from build123d import *

# Parameters (mm, degrees)
SKETCH1_R           = 1.8
BOSS_EXTRUDE1_DEPTH = 6
BOSS_EXTRUDE2_DEPTH = 40
CUT_EXTRUDE1_REACH  = 94.7
SKETCH3_W           = 20
SKETCH3_H           = 12.5
SKETCH4_R           = 3.25
CUT_EXTRUDE2_DEPTH  = 19
CUT_EXTRUDE3_REACH  = 102.286
CUT_EXTRUDE4_START  = -7
CUT_EXTRUDE4_DEPTH  = 26
SKETCH7_W           = 27
SKETCH7_H           = 36
CUT_EXTRUDE5_DEPTH  = 6
CUT_EXTRUDE6_REACH  = 95.13
SKETCH9_W           = 27
SKETCH9_H           = 32
CUT_EXTRUDE7_DEPTH  = 2
CUT_EXTRUDE10_DEPTH = 101.285841473
FILLET1_R           = 3
CUT_EXTRUDE11_DEPTH = 6
SKETCH12_W          = 8
SKETCH12_H          = 6
SKETCH12_W_2        = 10
BOSS_EXTRUDE3_DEPTH = 3
SKETCH13_R          = 2
CUT_EXTRUDE12_DEPTH = 6


with BuildPart() as part:
    # Sketch1 → Boss-Extrude1 (new body)
    with BuildSketch(Plane(origin=(0, 0, 0), x_dir=(1, 0, 0), z_dir=(0, 1, 0))):
        Polygon((68.5, 20), (68.5, 7.5), (88.5, 7.5), (88.5, -7.5), (68.5, -7.5), (68.5, -20), (-68.5, -20), (-68.5, -7.5), (-88.5, -7.5), (-88.5, 7.5), (-68.5, 7.5), (-68.5, 20), align=None)
        with Locations(Location((-78.5, 0, 0), (0, 0, 270))):
            Circle(SKETCH1_R, mode=Mode.SUBTRACT)
        with Locations(Location((-58.5, 8.5, 0), (0, 0, 270))):
            Circle(SKETCH1_R, mode=Mode.SUBTRACT)
        with Locations(Location((-58.5, -8.5, 0), (0, 0, 270))):
            Circle(SKETCH1_R, mode=Mode.SUBTRACT)
        with Locations(Location((58.5, -8.5, 0), (0, 0, 90))):
            Circle(SKETCH1_R, mode=Mode.SUBTRACT)
        with Locations(Location((78.5, 0, 0), (0, 0, 90))):
            Circle(SKETCH1_R, mode=Mode.SUBTRACT)
        with Locations(Location((58.5, 8.5, 0), (0, 0, 90))):
            Circle(SKETCH1_R, mode=Mode.SUBTRACT)
    extrude(amount=BOSS_EXTRUDE1_DEPTH)

    # Sketch2 → Boss-Extrude2 (add)
    with BuildSketch(Plane(origin=(0, 0, -20), x_dir=(-1, 0, 0), z_dir=(0, 0, -1))):
        Polygon((-88.5, 6), (88.5, 6), (88.5, 9), (58.5, 18), (48.5, 25), (-48.5, 25), (-58.5, 18), (-88.5, 9), align=None)
    extrude(amount=-BOSS_EXTRUDE2_DEPTH)

    # Sketch3 → Cut-Extrude1 (cut, up to next)
    with BuildSketch(Plane.XZ.offset(-6), mode=Mode.PRIVATE) as cut_extrude1_sk1:
        with Locations((-78.5, 13.75)):
            Rectangle(SKETCH3_W, SKETCH3_H)
    cut_extrude1_tool1 = extrude(cut_extrude1_sk1.sketch, amount=-CUT_EXTRUDE1_REACH, mode=Mode.PRIVATE) & part.part
    # Sketch3 → Cut-Extrude1 (cut, up to next)
    with BuildSketch(Plane.XZ.offset(-6), mode=Mode.PRIVATE) as cut_extrude1_sk2:
        with Locations((-78.5, -13.75)):
            Rectangle(SKETCH3_W, SKETCH3_H)
    cut_extrude1_tool2 = extrude(cut_extrude1_sk2.sketch, amount=-CUT_EXTRUDE1_REACH, mode=Mode.PRIVATE) & part.part
    # Sketch3 → Cut-Extrude1 (cut, up to next)
    with BuildSketch(Plane.XZ.offset(-6), mode=Mode.PRIVATE) as cut_extrude1_sk3:
        with Locations((78.5, 13.75)):
            Rectangle(SKETCH3_W, SKETCH3_H)
    cut_extrude1_tool3 = extrude(cut_extrude1_sk3.sketch, amount=-CUT_EXTRUDE1_REACH, mode=Mode.PRIVATE) & part.part
    # Sketch3 → Cut-Extrude1 (cut, up to next)
    with BuildSketch(Plane.XZ.offset(-6), mode=Mode.PRIVATE) as cut_extrude1_sk4:
        with Locations((78.5, -13.75)):
            Rectangle(SKETCH3_W, SKETCH3_H)
    cut_extrude1_tool4 = extrude(cut_extrude1_sk4.sketch, amount=-CUT_EXTRUDE1_REACH, mode=Mode.PRIVATE) & part.part
    add(cut_extrude1_tool1.solids().sort_by_distance((-78.5, 6, 13.75))[0], mode=Mode.SUBTRACT)
    add(cut_extrude1_tool2.solids().sort_by_distance((-78.5, 6, -13.75))[0], mode=Mode.SUBTRACT)
    add(cut_extrude1_tool3.solids().sort_by_distance((78.5, 6, 13.75))[0], mode=Mode.SUBTRACT)
    add(cut_extrude1_tool4.solids().sort_by_distance((78.5, 6, -13.75))[0], mode=Mode.SUBTRACT)

    # Sketch4 → Cut-Extrude2 (cut)
    with BuildSketch(Plane(origin=(0, 25, 0), x_dir=(1, 0, 0), z_dir=(0, 1, 0))):
        with Locations(Location((-58.5, 8.5, 0), (0, 0, 90))):
            Circle(SKETCH4_R)
        with Locations(Location((-78.5, 0, 0), (0, 0, 90))):
            Circle(SKETCH4_R)
        with Locations(Location((-58.5, -8.5, 0), (0, 0, 90))):
            Circle(SKETCH4_R)
        with Locations(Location((58.5, 8.5, 0), (0, 0, 90))):
            Circle(SKETCH4_R)
        with Locations(Location((58.5, -8.5, 0), (0, 0, 90))):
            Circle(SKETCH4_R)
        with Locations(Location((78.5, 0, 0), (0, 0, 180))):
            Circle(SKETCH4_R)
    extrude(amount=-CUT_EXTRUDE2_DEPTH, mode=Mode.SUBTRACT)

    # Sketch5 → Cut-Extrude3 (cut, up to next)
    with BuildSketch(Plane(origin=(0, 0, -20), x_dir=(-1, 0, 0), z_dir=(0, 0, -1)), mode=Mode.PRIVATE) as cut_extrude3_sk1:
        Polygon((48.5, 0), (30, 15), (-30, 15), (-48.5, 0), align=None)
    cut_extrude3_tool1 = extrude(cut_extrude3_sk1.sketch, amount=-CUT_EXTRUDE3_REACH, mode=Mode.PRIVATE) & part.part
    add(cut_extrude3_tool1.solids().sort_by_distance((0, 6.910828, -20))[0], mode=Mode.SUBTRACT)

    # Sketch6 → Cut-Extrude4 (cut)
    with BuildSketch(Plane(origin=(0, 0, -20), x_dir=(-1, 0, 0), z_dir=(0, 0, -1)).offset(CUT_EXTRUDE4_START)):
        Polygon((43.1, 4.378378378), (43.1, 20.378378378), (-53.9, 20.378378378), (-53.9, 0), (-48.5, 0), (-30, 15), (30, 15), align=None)
    extrude(amount=-CUT_EXTRUDE4_DEPTH, mode=Mode.SUBTRACT)

    # Sketch7 → Cut-Extrude5 (cut)
    with BuildSketch(Plane(origin=(0, 15, 0), x_dir=(-1, 0, 0), z_dir=(0, -1, 0))):
        with Locations((-5.5, 0)):
            Rectangle(SKETCH7_W, SKETCH7_H)
    extrude(amount=-CUT_EXTRUDE5_DEPTH, mode=Mode.SUBTRACT)

    # Sketch8 → Cut-Extrude6 (cut, up to next)
    with BuildSketch(Plane.XZ.offset(-21), mode=Mode.PRIVATE) as cut_extrude6_sk1:
        with BuildLine():
            Line((17, -18), (-6, -18))
            ThreePointArc((-6, -18), (-8, -16), (-6, -14))
            Line((-6, -14), (17, -14))
            ThreePointArc((17, -14), (19, -16), (17, -18))
        make_face()
    cut_extrude6_tool1 = extrude(cut_extrude6_sk1.sketch, amount=-CUT_EXTRUDE6_REACH, mode=Mode.PRIVATE) & part.part
    # Sketch8 → Cut-Extrude6 (cut, up to next)
    with BuildSketch(Plane.XZ.offset(-21), mode=Mode.PRIVATE) as cut_extrude6_sk2:
        with BuildLine():
            Line((17, 14), (-6, 14))
            ThreePointArc((-6, 14), (-8, 16), (-6, 18))
            Line((-6, 18), (17, 18))
            ThreePointArc((17, 18), (19, 16), (17, 14))
        make_face()
    cut_extrude6_tool2 = extrude(cut_extrude6_sk2.sketch, amount=-CUT_EXTRUDE6_REACH, mode=Mode.PRIVATE) & part.part
    add(cut_extrude6_tool1.solids().sort_by_distance((5.5, 21, -16))[0], mode=Mode.SUBTRACT)
    add(cut_extrude6_tool2.solids().sort_by_distance((5.5, 21, 16))[0], mode=Mode.SUBTRACT)

    # Sketch9 → Cut-Extrude7 (cut)
    with BuildSketch(Plane(origin=(0, 25, 0), x_dir=(1, 0, 0), z_dir=(0, 1, 0))):
        with Locations((5.5, 0)):
            Rectangle(SKETCH9_W, SKETCH9_H)
    extrude(amount=-CUT_EXTRUDE7_DEPTH, mode=Mode.SUBTRACT)

    # Sketch10 → Cut-Extrude10 (cut, through all)
    with BuildSketch(Plane(origin=(0, 0, -20), x_dir=(-1, 0, 0), z_dir=(0, 0, -1))):
        Polygon((43.1, 4.378378378), (30, 15), (43.1, 15), align=None)
    extrude(amount=-CUT_EXTRUDE10_DEPTH, mode=Mode.SUBTRACT)

    # Fillet1
    fillet1_edges = [part.edges().sort_by_distance(p)[0] for p in [
        (-43.1, 15, -16.5),
        (-43.1, 15, 16.5),
    ]]
    fillet(fillet1_edges, radius=FILLET1_R)

    # Sketch11 → Cut-Extrude11 (cut)
    with BuildSketch(Plane.XY.offset(20)):
        Polygon((25.5, 25), (48.5, 25), (58.5, 18), (68.5, 15), (68.5, 3), (52.633333333, 3), align=None)
        with BuildLine():
            Line((-68.5, 3), (-47.7, 3))
            Line((-47.7, 3), (-47.7, 13.5))
            ThreePointArc((-47.7, 13.5), (-46.528427125, 16.328427125), (-43.7, 17.5))
            Line((-43.7, 17.5), (-23.75, 17.5))
            Line((-23.75, 17.5), (-14.5, 25))
            Line((-14.5, 25), (-48.5, 25))
            Line((-48.5, 25), (-58.5, 18))
            Line((-58.5, 18), (-68.5, 15))
            Line((-68.5, 15), (-68.5, 3))
        make_face()
    cut_extrude11 = extrude(amount=-CUT_EXTRUDE11_DEPTH, mode=Mode.SUBTRACT)

    # Mirror1: Cut-Extrude11 across plane
    add(cut_extrude11.mirror(Plane(origin=(0, 0, 0), x_dir=(1, 0, 0), z_dir=(0, 0, -1))), mode=Mode.SUBTRACT)

    # Sketch12 → Boss-Extrude3 (add)
    with BuildSketch(Plane(origin=(0, 3, 0), x_dir=(1, 0, 0), z_dir=(0, 1, 0))):
        with Locations((-51.7, 17)):
            Rectangle(SKETCH12_W, SKETCH12_H)
        with Locations((-51.7, -17)):
            Rectangle(SKETCH12_W, SKETCH12_H)
        with Locations((53.5, -17)):
            Rectangle(SKETCH12_W_2, SKETCH12_H)
        with Locations((53.5, 17)):
            Rectangle(SKETCH12_W_2, SKETCH12_H)
    extrude(amount=BOSS_EXTRUDE3_DEPTH)

    # Sketch13 → Cut-Extrude12 (cut)
    with BuildSketch(Plane(origin=(0, 6, 0), x_dir=(1, 0, 0), z_dir=(0, 1, 0))):
        with Locations(Location((54.5, -17, 0), (0, 0, 270))):
            Circle(SKETCH13_R)
        with Locations(Location((54.5, 17, 0), (0, 0, 270))):
            Circle(SKETCH13_R)
        with Locations(Location((-51.7, 17, 0), (0, 0, 270))):
            Circle(SKETCH13_R)
        with Locations(Location((-51.7, -17, 0), (0, 0, 270))):
            Circle(SKETCH13_R)
    extrude(amount=-CUT_EXTRUDE12_DEPTH, mode=Mode.SUBTRACT)


solid = part.part
CAD build for the part. Positions are in the model's coordinates, mm. A direction names the side the tool comes from. Give positions to 0.01 mm unless a question says otherwise; leave off trailing zeros. Loops run counter-clockwise (first coordinate to the right, second up) from the corner with the lowest first, then second, coordinate; pieces in that order, holes last. Notation, with made-up numbers: M 16.25,-26 L 43.25,-26 A26 ccw 43.25,-11 Z; hole C -17.5,67 d10. An arc over 180 degrees is marked long. Write each question's results on one line, items separated by ' | '.
Q1. Probe probe 1 along X at (y, z) = (8, 0); probe 2 along X at (y, z) = (14.5, 8.5); probe 3 along Z at (x, y) = (-78.5, 1.55). List the from-to ranges inside material, lowest first.
Geometry check:
probe 1: x = -88.5 to -81.75, -75.25 to -43.1, 53.9 to 75.25, 81.75 to 88.5 | probe 2: x = -68.5 to -61.75, -55.25 to -43.1, 53.9 to 55.25, 61.75 to 68.5 | probe 3: z = -7.5 to -1.8, 1.8 to 7.5
Q2. Band-saw the part on A-A on x = -78.5. Write the cut outline in (y, z).
Geometry check:
outline: M 0,-7.5 L 12,-7.5 L 12,-3.25 L 6,-3.25 L 6,-1.8 L 0,-1.8 Z; M 0,1.8 L 6,1.8 L 6,3.25 L 12,3.25 L 12,7.5 L 0,7.5 Z
Q3. Flat gauge pins, fed straight in: P1, Ø1.5, axis at y = 5, z = -16.5, coming from the +X side; P2, Ø5, axis at x = -52, z = -17, coming from the +Y side; P3, Ø2, axis at x = 32.5, y = 11, coming from the +Z side; P4, Ø3, axis at x = 64, z = -11.5, coming from the +Y side. Where does each tip first touch, or does it go through?
Geometry check:
P1: stops at x = 58.5 | P2: stops at y = 6 | P3: passes through | P4: stops at y = 16.8
Q4. Mould opens along Z. For faces 6 (the face through (39.12, 7.605, -16.549)), 7 (the face through (0.3, 15.3, 20)), 8 (the face through (55.278, 11.671, 8.923)) say: pulls with the +Z half, pulls with the -Z half, needs draft (parallel to the pull), parting line crosses it, or undercut.
Geometry check:
face 6: needs draft | face 7: pulls with the +Z half | face 8: undercut
Q5. Which spindle directions (+Z, -Z, +X, -X, +Y, -Y) get a long thin tool onto all of the face, cutting with end or side? Do faces 1 (the face through (-12, 15, -17)), 2 (the face through (60, 6, 7)), 3 (the face through (41, 13, -13)), 4 (the face through (-34, 17.5, -17)), 5 (the face through (-46.559, 16.297, 17.042)). Say none if no direction does.
Geometry check:
face 1: +Z, -Z, -Y | face 2: +Y | face 3: -Y | face 4: -Z, -X, +Y | face 5: +Z, -X, +Y
Q6. Band-saw the part on D-D on z = 0. Give the number of separate pieces and of enclosed holes in the cut face, and give its area (3 significant figures).
Geometry check:
separate pieces: 3 | enclosed holes: 0 | area: 1,480 mm²
Q7. Band-saw the part on B-B on x = 5. Write the cut outline in (y, z).
Geometry check:
outline: M 15,-20 L 25,-20 L 25,-18 L 15,-18 Z; M 15,18 L 25,18 L 25,20 L 15,20 Z; M 21,-14 L 23,-14 L 23,14 L 21,14 Z
Q8. Band-saw the part on C-C on x = 67. Write the cut outline in (y, z), and give its area (3 significant figures).
Geometry check:
outline: M 0,-20 L 3,-20 L 3,-14 L 15.45,-14 L 15.45,14 L 3,14 L 3,20 L 0,20 Z | area: 469 mm²
